Design review of the part shown in the three views and the two pictorial views. Dimensions are in mm from the part's minimum x, y and z. A direction names the side the tool comes from. Round coordinates to 2 decimals unless told otherwise and drop trailing zeros. Order: outer loops, then holes, each group sorted by start corner. A loop starts at its lowest first (then second) coordinate and runs counter-clockwise, first axis right, second up.
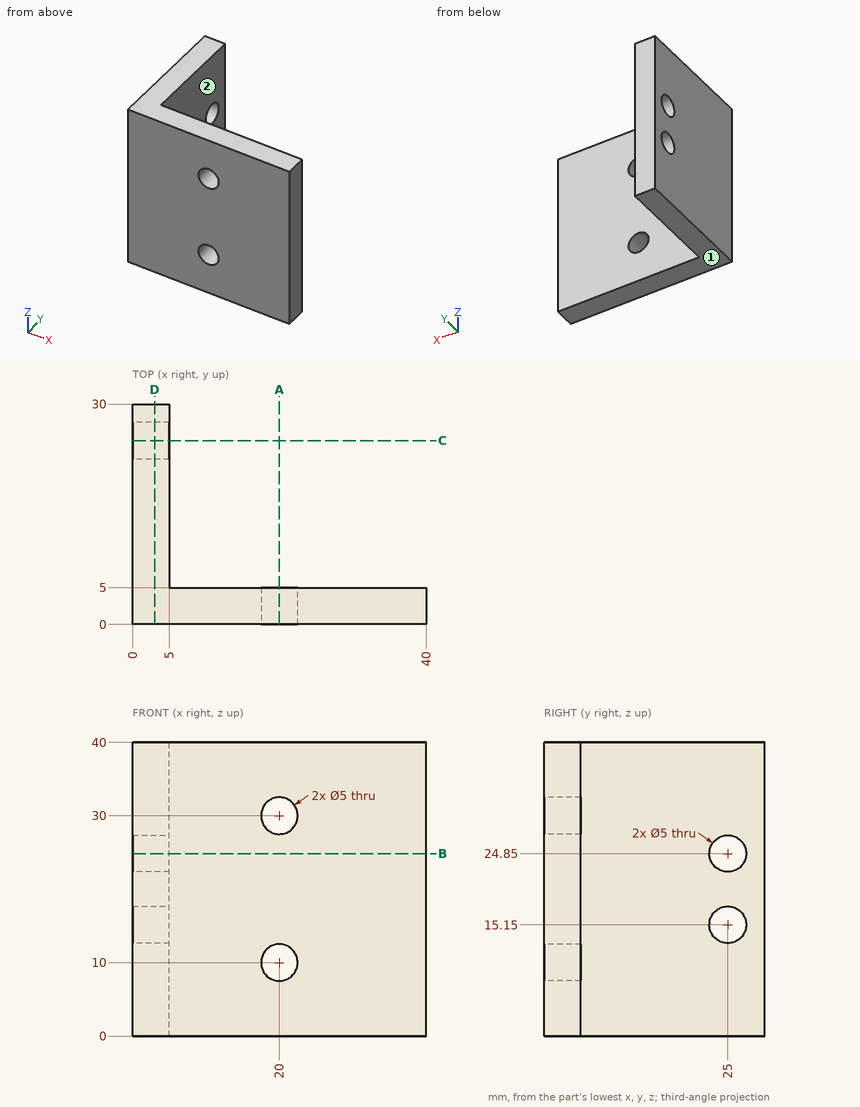
(1) Clearance check with a flat-ended pin moving along its axis: P1, Ø1.5, axis at y = 7.5, z = 18, coming from the +X side. State where the tip first meets the part, or that it passes through.
(2) Add section A-A on x = 20. Give the boundary of the cut face in (y, z).
(3) Tool access review of the marked faces 1 and 2: name each direction out of +Z, -Z, +X, -X, +Y, -Y from which nothing blocks a thin tool from reaching the whole face with its end or side.
(4) Add section B-B on z = 24.85. Give the boundary of the cut face in (x, y), plus the area to 3 significant figures.
(5) Add section C-C on y = 25. Give the boundary of the cut face in (x, z), plus the area to 3 significant figures.
(6) Add section D-D on x = 3. Give the boundary of the cut face in (y, z), plus the area to 3 significant figures.
(7) Wall thickness on L1, parallel to Z at x = 20, y = 1.75; L2, parallel to Y at x = 28, z = 8.5; L3, parallel to Y at x = 3, z = 15.15: over which ranges is each line inside the solid? List them lowest first.
Here are the results:
1. P1: stops at x = 5
2. outline: (0, 0) - (5, 0) - (5, 7.5) - (0, 7.5) - close; (0, 12.5) - (5, 12.5) - (5, 27.5) - (0, 27.5) - close; (0, 32.5) - (5, 32.5) - (5, 40) - (0, 40) - close
3. face 1: -Z, +X, -X, +Y, -Y
3. face 2: +Z, -Z, +X, +Y
4. outline: (0, 0) - (40, 0) - (40, 5) - (5, 5) - (5, 22.5) - (0, 22.5) - close; (0, 27.5) - (5, 27.5) - (5, 30) - (0, 30) - close
4. area: 300 mm2
5. outline: (0, 0) - (5, 0) - (5, 12.65) - (0, 12.65) - close; (0, 17.65) - (5, 17.65) - (5, 22.35) - (0, 22.35) - close; (0, 27.35) - (5, 27.35) - (5, 40) - (0, 40) - close
5. area: 150 mm2
6. outline: (0, 0) - (30, 0) - (30, 40) - (0, 40) - close; hole circle Ø5 at (25, 15.15); hole circle Ø5 at (25, 24.85)
6. area: 1,160 mm2
7. L1: z = 0 to 7.5, 12.5 to 27.5, 32.5 to 40
7. L2: y = 0 to 5
7. L3: y = 0 to 22.5, 27.5 to 30
